Design review of the part built by this model. Coordinates are the model's own, in mm. Face numbers are marked on the shaded views. A direction names the side the tool comes from. Give positions to 0.01 mm unless a question says otherwise; leave off trailing zeros. Write each loop counter-clockwise with the first axis right and the second up, starting at its lowest first coordinate (ties: lowest second). Pieces come first, ordered by that corner, then holes. Notation, with made-up numbers: M -35,33.5 L 19,33.5 A7 cw 19,42.5 Z; hole C 72.5,-14 d3. An arc over 180 degrees is marked long. Answer in a Markdown table with one row per item.
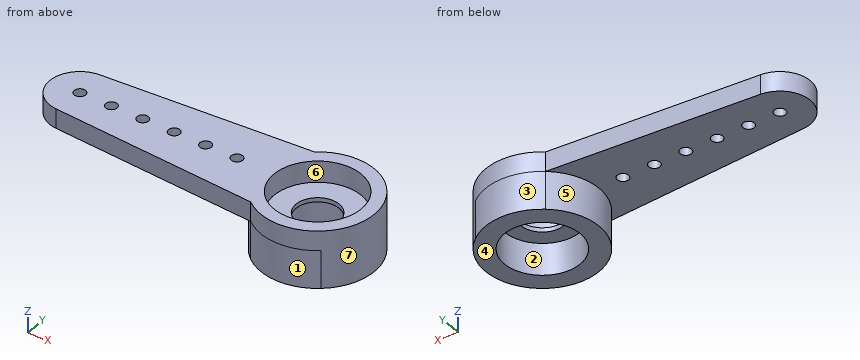
Autodesk Inventor part; units mm, degrees
ref_plane "YZ Plane" through (0, 0, 0) normal (1, 0, 0) x (0, 1, 0)
ref_plane "XZ Plane" through (0, 0, 0) normal (0, 1, 0) x (-1, 0, 0)
ref_plane "XY Plane" through (0, 0, 0) normal (0, 0, 1) x (1, 0, 0)
sketch "Sketch1" plane through (0, 0, 0) normal (0, 0, 1) x (1, 0, 0)
  circle A0 centre (0, 0) radius 3.4036
  circle A1 centre (-14.4145, 0) radius 1.8161
  circle A2 centre (14.4145, 0) radius 1.8161
  line L0 (0, 0) -> (0, 12.9246) construction
  line L1 (-14.5375, 1.8119) -> (-2.1305, 2.6543)
  line L2 (2.1305, 2.6543) -> (14.5375, 1.8119)
  line L3 (14.5375, -1.8119) -> (2.1305, -2.6543)
  line L4 (-2.1305, -2.6543) -> (-14.5375, -1.8119)
  dimension "d0" = 6.8072
  dimension "d1" = 3.6322
  dimension "d2" = 32.4612
  dimension "d3" = 5.3086
extrude "Extrusion1" add sketch "Sketch1" along normal blind 1.1684
sketch "Sketch2" plane through (0, 0, 0) normal (0, 0, -1) x (-1, 0, 0)
  arc A0 (14.5375, -1.8119) -> (14.5375, 1.8119) centre (14.4145, 0) ccw
  line L0 (2.1305, 2.6543) -> (14.5375, 1.8119)
  arc A1 (2.1305, 2.6543) -> (-2.1305, 2.6543) centre (0, 0) ccw
  line L1 (-14.5375, 1.8119) -> (-2.1305, 2.6543)
  arc A2 (-14.5375, 1.8119) -> (-14.5375, -1.8119) centre (-14.4145, 0) ccw
  line L2 (-2.1305, -2.6543) -> (-14.5375, -1.8119)
  arc A3 (-2.1305, -2.6543) -> (2.1305, -2.6543) centre (0, 0) ccw
  line L3 (14.5375, -1.8119) -> (2.1305, -2.6543)
  circle A4 centre (0, 0) radius 3.4036
extrude "Extrusion2" add sketch "Sketch2" along normal blind 2.2606 contours A3 A4 A1
sketch "Sketch3" plane through (0, 0, -2.2606) normal (0, 0, -1) x (-1, 0, 0)
  circle A0 centre (0, 0) radius 2.2733
  dimension "d8" = 4.5466
extrude "Extrusion3" cut sketch "Sketch3" against normal blind 1.905
sketch "Sketch4" plane through (0, 0, 1.1684) normal (0, 0, 1) x (1, 0, 0)
  circle A0 centre (0, 0) radius 2.6162
  dimension "d11" = 5.2324
extrude "Extrusion4" cut sketch "Sketch4" against normal blind 1.27
sketch "Sketch5" plane through (0, 0, -0.1016) normal (0, 0, 1) x (1, 0, 0)
  circle A0 centre (0, 0) radius 1.2954
  dimension "d14" = 2.5908
extrude "Extrusion5" cut sketch "Sketch5" against normal blind 1.27
sketch "Sketch6" plane through (0, 0, 1.1684) normal (0, 0, 1) x (1, 0, 0)
  arc A0 (-14.5375, 1.8119) -> (-14.5375, -1.8119) centre (-14.4145, 0) ccw
  circle A1 centre (-14.4145, 0) radius 0.3429
  point P0 (0, 0)
  dimension "d17" = 0.6858
extrude "Extrusion6" cut sketch "Sketch6" against normal through all
pattern_linear "Rectangular Pattern1" count 6 spacing 1.905 along (1, 0, 0) of "Extrusion6"
mirror "Mirror1" about plane through (0, 0, 0) normal (1, 0, 0) of "Extrusion6", "Rectangular Pattern1"
sketch "Sketch7" plane through (0, 0, 1.1684) normal (0, 0, 1) x (1, 0, 0)
  arc A0 (2.1305, 2.6543) -> (-2.1305, 2.6543) centre (0, 0) ccw
  arc A1 (-2.1305, -2.6543) -> (2.1305, -2.6543) centre (0, 0) ccw
  circle A2 centre (0, 0) radius 3.4036
  circle A3 centre (0, 0) radius 3.4036
  line L0 (1.1266, 3.2117) -> (19.4496, 9.8398)
  line L1 (19.4496, 9.8398) -> (21.7312, -12.9756)
  line L2 (21.7312, -12.9756) -> (1.4617, -3.0737)
extrude "Extrusion7" cut sketch "Sketch7" against normal through all contours A0 L0 L1 L2 A1 A2
properties part number "1 Way MicroServo Attachment"
1) To check wall thickness, follow probe 1 along Z at (x, y) = (-7, -1); probe 2 along Y at (x, z) = (-1, 0.7); probe 3 along Y at (x, z) = (-0.25, -0.3). State the ranges of each line that lie inside material, in increasing order. Write a range as [from, to].
Geometry says:
| item | result |
|---|---|
| probe 1 | [0, 1.17] |
| probe 2 | [-3.25, -2.42], [2.42, 3.25] |
| probe 3 | [-3.39, -1.27], [1.27, 3.39] |
2) For the marked faces 5, 6 and 7, list the 3-axis set-ups (+Z, -Z, +X, -X, +Y, -Y) from which the entire face can be reached by the end or side of a thin tool; tool diameter is ignored.
Geometry says:
| item | result |
|---|---|
| face 5 | -Z, -X |
| face 6 | +Z |
| face 7 | +Z, -Z |
3) Add section C-C (y = 0). Count the separate pieces of the cut face and the enclosed holes in it, and give its area (3 significant figures).
Geometry says:
| item | result |
|---|---|
| separate pieces | 8 |
| enclosed holes | 0 |
| area | 17.6 mm^2 |
4) Add section D-D (z = -0.9). Write out the cut boundary in (x, y), and give its area (3 significant figures).
Geometry says:
| item | result |
|---|---|
| outline | M -2.13,-2.65 A3.4 ccw 2.13,-2.65 A3.4 ccw long Z; hole C 0,0 d4.55 |
| area | 20.2 mm^2 |
5) Add section B-B (x = 0). Write out the cut boundary in (y, z), and give its area (3 significant figures).
Geometry says:
| item | result |
|---|---|
| outline | M -3.4,-2.26 L -2.27,-2.26 L -2.27,-0.36 L -1.3,-0.36 L -1.3,-0.1 L -2.62,-0.1 L -2.62,1.17 L -3.4,1.17 Z; M 1.3,-0.36 L 2.27,-0.36 L 2.27,-2.26 L 3.4,-2.26 L 3.4,1.17 L 2.62,1.17 L 2.62,-0.1 L 1.3,-0.1 Z |
| area | 7.38 mm^2 |
6) The part is to be moulded in two halves that separate along Y. For the marked faces 1, 2, 3 and 4, say which applies: released by +Y, released by -Y, zero draft, split by the parting line, or undercut.
Geometry says:
| item | result |
|---|---|
| face 1 | released by -Y |
| face 2 | undercut |
| face 3 | released by +Y |
| face 4 | zero draft |
7) Add section A-A (z = 0.95). Write out the cut boundary in (x, y), and give its area (3 significant figures).
Geometry says:
| item | result |
|---|---|
| outline | M -14.54,-1.81 L -2.13,-2.65 A3.4 ccw long -2.13,2.65 L -14.54,1.81 A1.82 ccw Z; hole C -14.41,0 d0.69; hole C -12.51,0 d0.69; hole C -10.6,0 d0.69; hole C -8.7,0 d0.69; hole C -6.79,0 d0.69; hole C -4.89,0 d0.69; hole C 0,0 d5.23 |
| area | 68.1 mm^2 |
8) Insertion check: P1, Ø3.5, axis at x = 0, y = 0, coming from the +Z side; P2, Ø2, axis at x = 1.5, z = -1.5, coming from the -Y side; P3, Ø1.4, axis at x = 0, y = -1, coming from the -Z side. Each pin has a flat end and moves straight along its axis. Give the tip position at first contact, or say it passes through.
Geometry says:
| item | result |
|---|---|
| P1 | z = -0.1 |
| P2 | y = -3.37 |
| P3 | z = -0.36 |
